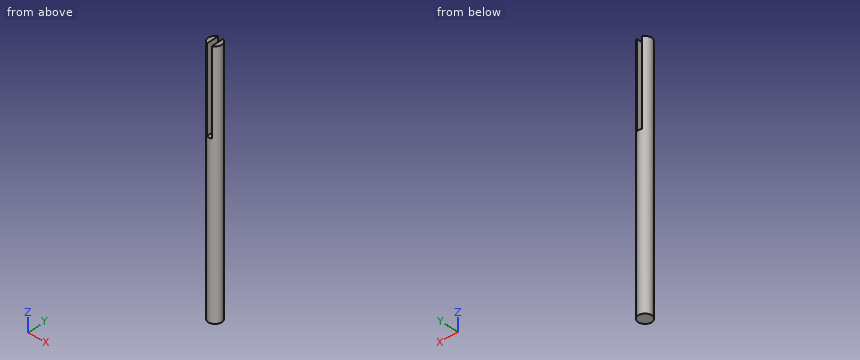
Autodesk Inventor part; units mm, degrees
ref_plane "YZ Plane" through (0, 0, 0) normal (1, 0, 0) x (0, 1, 0)
ref_plane "XZ Plane" through (0, 0, 0) normal (0, 1, 0) x (-1, 0, 0)
ref_plane "XY Plane" through (0, 0, 0) normal (0, 0, 1) x (1, 0, 0)
sketch "Sketch1" plane through (0, 0, 0) normal (0, 0, 1) x (1, 0, 0)
  circle A0 centre (0, 0) radius 4.05
  circle A1 centre (0, 0) radius 7.5
  circle A2 centre (0, 0) radius 4.05
  circle A3 centre (0, 0) radius 4
  dimension "d0" = 8
extrude "Extrusion1" add sketch "Sketch1" along normal blind 100 contours A3
sketch "Sketch2" plane through (0, 0, 100) normal (0, 0, 1) x (1, 0, 0)
  circle A0 centre (0, 0) radius 4
  line L0 (-1.5, 4) -> (-1.5, -4)
  line L1 (-1.5, -4) -> (1.5, -4)
  line L2 (1.5, -4) -> (1.5, 4)
  line L3 (1.5, 4) -> (-1.5, 4)
  line L4 (-1.5, 4) -> (1.5, -4) construction
  line L5 (-1.5, -4) -> (1.5, 4) construction
  point P0 (-1.5, -3.7081)
  point P1 (-1.5, 3.7081)
  point P2 (1.5, 3.7081)
  point P3 (1.5, -3.7081)
  dimension "d3" = 3
extrude "Extrusion2" add sketch "Sketch2" along normal blind 50 contours A0 L2 | L0 A0
properties part number "spirale"
Design review of the part built by this model. Coordinates are the model's own, in mm. Coordinates: 2 decimals unless noted, no trailing zeros. Loops run counter-clockwise (first coordinate to the right, second up) from the corner with the lowest first, then second, coordinate; pieces in that order, holes last.
Item 1: Wall thickness on L1, parallel to X at y = 1.5, z = 28; L2, parallel to Z at x = -1, y = 1.5; L3, parallel to X at y = -2.25, z = 128.5: over which ranges is each line inside the solid? List them lowest first.
Completed:
L1: x = -3.71 to 3.71
L2: z = 0 to 100
L3: x = -3.31 to -1.5, 1.5 to 3.31
Item 2: Add section A-A (y = -1.5). Write out the cut boundary in (x, z).
Completed:
outline: (-3.71, 0) - (3.71, 0) - (3.71, 150) - (1.5, 150) - (1.5, 100) - (-1.5, 100) - (-1.5, 150) - (-3.71, 150) - close
Item 3: Clearance check with flat-ended pins moving along their axes: pin 1 (2.5 mm diameter, centred on x = 0, y = 0, fed in from +Z); pin 2 (1.5 mm diameter, centred on x = -2.5, z = 113, fed in from -Y). State where each tip first meets the part, or that it passes through.
Completed:
pin 1: stops at z = 100
pin 2: stops at y = -3.6
Item 4: Add section B-B (x = 0). Write out the cut boundary in (y, z), and give its area (3 significant figures).
Completed:
outline: (-4, 0) - (4, 0) - (4, 100) - (-4, 100) - close
area: 800 mm2
Item 5: Add section C-C (z = 54). Write out the cut boundary in (x, y), and give its area (3 significant figures).
Completed:
outline: circle Ø8 at (0, 0)
area: 50.3 mm2
